Source: three-view drawing plus pictorial views. Frame: mm from the lowest corner of the part. Coordinates: 2 decimals unless noted, no trailing zeros. Loops run counter-clockwise (first coordinate to the right, second up) from the corner with the lowest first, then second, coordinate; pieces in that order, holes last.
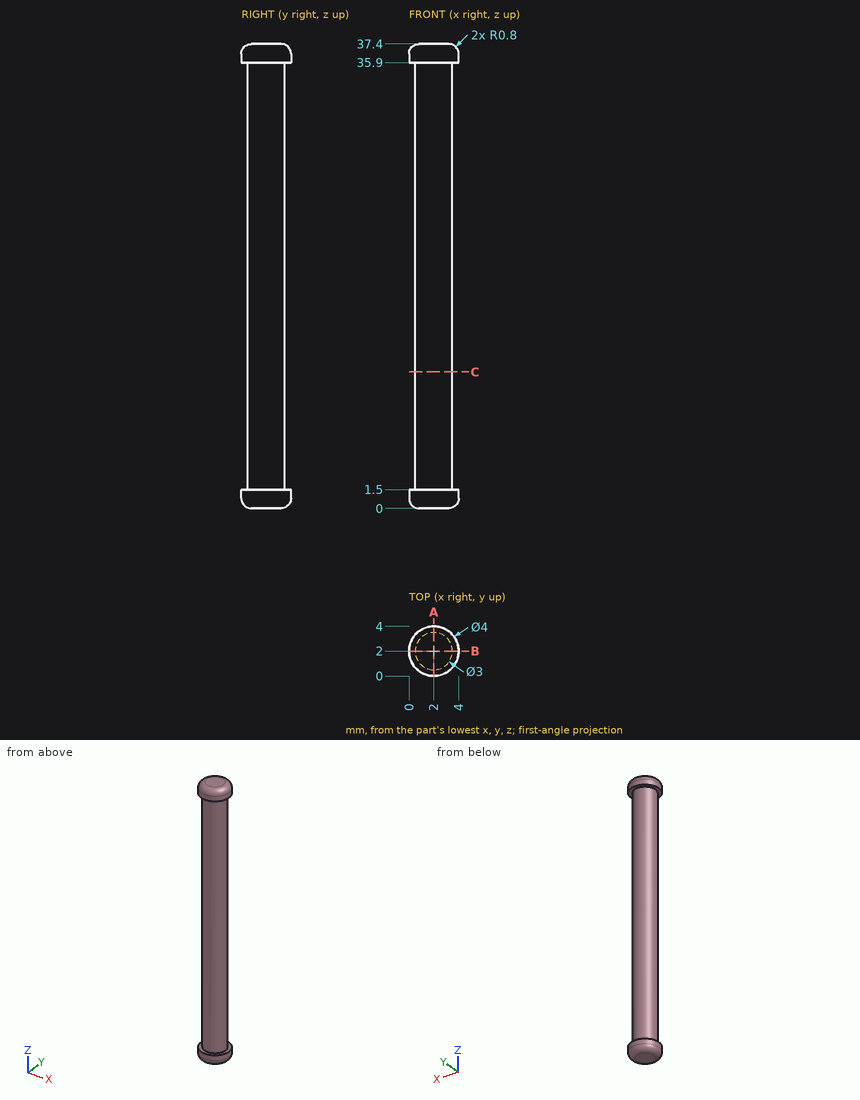
Q1. Section query A-A on x = 2. Return the cut outline in (y, z), then the cut area to 3 significant figures.
Q2. Section query C-C on z = 11. Return the cut outline in (x, y).
Q3. First-contact query: pin 1 Ø1.5 at (y, z) = (0.5, 21) entering from +X; pin 2 Ø2 at (x, z) = (3, 18.5) entering from +Y. Flat tips, straight axial feed; report the tip coordinate or a pass-through.
Q4. Material intervals for line 1 along Y through (x, z) = (2.05, 4); line 2 along Z through (x, y) = (3.3, 1.2); line 3 along Z through (x, y) = (0.65, 3), sorted ascending.
Resolved:
1. outline: (0, 0.8) arc R0.8 ccw to (0.8, 0) - (3.2, 0) arc R0.8 ccw to (4, 0.8) - (4, 1.5) - (3.5, 1.5) - (3.5, 35.9) - (4, 35.9) - (4, 36.6) arc R0.8 ccw to (3.2, 37.4) - (0.8, 37.4) arc R0.8 ccw to (0, 36.6) - (0, 35.9) - (0.5, 35.9) - (0.5, 1.5) - (0, 1.5) - close
1. area: 115 mm2
2. outline: circle Ø3 at (2, 2)
3. pin 1: stops at x = 3.3
3. pin 2: stops at y = 3.5
4. line 1: y = 0.5 to 3.5
4. line 2: z = 0.07 to 1.5, 35.9 to 37.33
4. line 3: z = 0.16 to 1.5, 35.9 to 37.24
